Part model, mm, in its own coordinate system. Face numbers are marked on the shaded views. A direction names the side the tool comes from. Round coordinates to 2 decimals unless told otherwise and drop trailing zeros. Write each loop counter-clockwise with the first axis right and the second up, starting at its lowest first coordinate (ties: lowest second). Pieces come first, ordered by that corner, then holes. Notation, with made-up numbers: M 75,41.5 L 111,41.5 A17 ccw 111,67.5 Z; hole C 52,53 d3. An arc over 180 degrees is marked long. Answer as a JSON object with one key per item and string values. Group by question number.
1. Drill centre lines: line 1 (X direction, y = 2.6, z = 0); line 2 (Z direction, x = 0, y = 7.5); line 3 (X direction, y = 1.1, z = 0). Where is each one in solid material? Low to high. Write a range as from..to.
2. Drop flat-ended pins along their axis: pin 1 (2 mm diameter, centred on x = -7, z = -41.5, fed in from +Y); pin 2 (22.5 mm diameter, centred on x = 5, z = 6, fed in from +Y); pin 3 (6 mm diameter, centred on y = 2, z = -41.5, fed in from -X). Give the stop position or say it passes through.
3. Two-plate mould, pull along X, no slides. Class the marked faces 3, 4 and 5: +X half, -X half, draft (parallel to the pull), parting line (faces both ways), or undercut.
4. Band-saw the part on C-C, the plane y = 7.5. Write the cut outline in (x, z), plus the area to 3 significant figures.
5. Which spindle directions (+Z, -Z, +X, -X, +Y, -Y) get a long thin tool onto all of the face, cutting with end or side? Do the marked faces 1 and 2. Say none if no direction does.
from build123d import *

# Parameters (mm, degrees)
SKETCH1_R            = 53.5
BOSS_EXTRUDE1_DEPTH  = 19
SKETCH2_R            = 49.5
CUT_EXTRUDE1_DEPTH   = 6
FILLET1_R            = 2
SKETCH3_R            = 14
BOSS_EXTRUDE2_DEPTH  = 4
FILLET2_R            = 2
FILLET1_OF_MIRROR1_R = 2
FILLET2_OF_MIRROR1_R = 2
SKETCH5_R            = 6
CUT_EXTRUDE2_DEPTH   = 18


with BuildPart() as part:
    # Sketch1 → Boss-Extrude1 (new body)
    with BuildSketch(Plane(origin=(0, 0, 0), x_dir=(1, 0, 0), z_dir=(0, 1, 0))):
        Circle(SKETCH1_R)
    extrude(amount=BOSS_EXTRUDE1_DEPTH)

    # Sketch2 → Cut-Extrude1 (cut)
    with BuildSketch(Plane(origin=(0, 19, 0), x_dir=(1, 0, 0), z_dir=(0, 1, 0))):
        Circle(SKETCH2_R)
    cut_extrude1 = extrude(amount=-CUT_EXTRUDE1_DEPTH, mode=Mode.SUBTRACT)

    # Fillet1
    fillet1_edges = [part.edges().sort_by_distance(p)[0] for p in [
        (-49.5, 13, 0),
    ]]
    fillet(fillet1_edges, radius=FILLET1_R)

    # Sketch3 → Boss-Extrude2 (add)
    with BuildSketch(Plane(origin=(0, 13, 0), x_dir=(1, 0, 0), z_dir=(0, 1, 0))):
        Circle(SKETCH3_R)
    boss_extrude2 = extrude(amount=BOSS_EXTRUDE2_DEPTH)

    # Fillet2
    fillet2_edges = [part.edges().sort_by_distance(p)[0] for p in [
        (-14, 13, 0),
    ]]
    fillet(fillet2_edges, radius=FILLET2_R)

    # Mirror1: Cut-Extrude1, Boss-Extrude2 across plane
    add(cut_extrude1.mirror(Plane.ZX.offset(9.5)), mode=Mode.SUBTRACT)
    add(boss_extrude2.mirror(Plane.ZX.offset(9.5)))

    # Fillet1 of Mirror1
    fillet1_of_mirror1_edges = [part.edges().sort_by_distance(p)[0] for p in [
        (-49.5, 6, 0),
    ]]
    fillet(fillet1_of_mirror1_edges, radius=FILLET1_OF_MIRROR1_R)

    # Fillet2 of Mirror1
    fillet2_of_mirror1_edges = [part.edges().sort_by_distance(p)[0] for p in [
        (-14, 6, 0),
    ]]
    fillet(fillet2_of_mirror1_edges, radius=FILLET2_OF_MIRROR1_R)

    # Sketch5 → Cut-Extrude2 (cut, through all)
    with BuildSketch(Plane(origin=(0, 17, 0), x_dir=(1, 0, 0), z_dir=(0, 1, 0))):
        Circle(SKETCH5_R)
    extrude(amount=-CUT_EXTRUDE2_DEPTH, mode=Mode.SUBTRACT)


solid = part.part
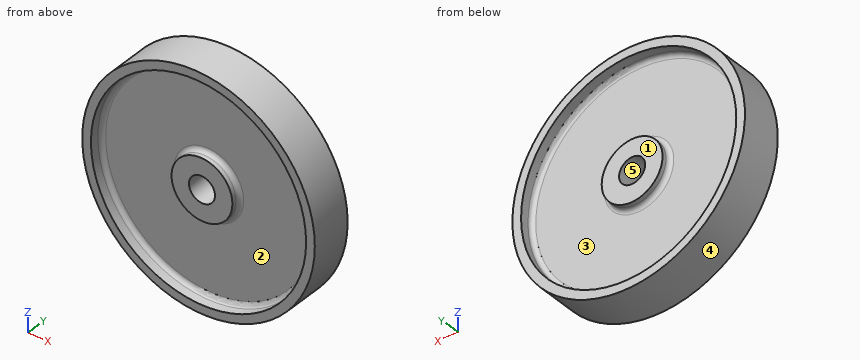
Worked answers:
{
 "1": {"line 1": "x = -53.5..-49.5, -14..-6, 6..14, 49.5..53.5", "line 2": "z = -53.5..-6, 6..53.5", "line 3": "x = -53.5..-49.5, 49.5..53.5"},
 "2": {"pin 1": "stops at y = 13", "pin 2": "stops at y = 17", "pin 3": "stops at x = -37.15"},
 "3": {"face 3": "undercut", "face 4": "parting line", "face 5": "undercut"},
 "4": {"outline": "C 0,0 d107; hole C 0,0 d12", "area": "8,880 mm^2"},
 "5": {"face 1": "+Y", "face 2": "-Y"}
}
